Geometry check sheet. Reference: the model listing, model coordinates, mm. A direction names the side the tool comes from. Coordinates: 2 decimals unless noted, no trailing zeros. Loops run counter-clockwise (first coordinate to the right, second up) from the corner with the lowest first, then second, coordinate; pieces in that order, holes last.
Autodesk Inventor part; units mm, degrees
sketch "Эскиз1" plane through (0, 0, 0) normal (0, 0, 1) x (1, 0, 0)
  line L0 (-29.5, -27.5) -> (29.5, -27.5)
  line L1 (29.5, -27.5) -> (29.5, 27.5)
  line L2 (29.5, 27.5) -> (-29.5, 27.5)
  line L3 (-29.5, 27.5) -> (-29.5, -27.5)
  line L4 (-29.5, -27.5) -> (29.5, 27.5) construction
  line L5 (29.5, -27.5) -> (-29.5, 27.5) construction
  line L6 (0, -7.5) -> (0, -27.5) construction
  circle A0 centre (-21.05, 22.5) radius 1.5
  circle A1 centre (21.05, 22.5) radius 1.5
  line L7 (-21.05, 22.5) -> (21.05, 22.5)
  point P0 (0, 0)
  dimension "d0" = 59
  dimension "d1" = 55
  dimension "d3" = 20
  dimension "d4" = 3
  dimension "d7" = 42.1
  dimension "d8" = 8.45
  dimension "d13" = 5
extrude "Выдавливание1" add sketch "Эскиз1" along normal blind 4
sketch "Эскиз2" plane through (0, 0, 4) normal (0, 0, 1) x (1, 0, 0)
  line L0 (29.5, 27.5) -> (-29.5, 27.5)
  line L1 (-2.5247, 27.5) -> (-2.5247, 11.5)
  line L2 (2.5247, 27.5) -> (2.5247, 11.5)
  line L3 (-2.5247, 11.5) -> (2.5247, 11.5)
  point P0 (0, 0)
  dimension "d9" = 16
extrude "Выдавливание2" cut sketch "Эскиз2" against normal up to surface (4 mm away)
fillet "Сопряжение1" radius 2 4 edges at (2.5247, 11.5, 2) (-2.5247, 11.5, 2) (2.5247, 27.5, 2) (-2.5247, 27.5, 2)
sketch "Эскиз3" plane through (0, 0, 4) normal (0, 0, 1) x (1, 0, 0)
  line L0 (-29.5, 27.5) -> (-29.5, -27.5)
  line L1 (-29.5, -17.5) -> (-19.5, -17.5) construction
  line L2 (-19.5, -17.5) -> (-19.5, -27.5) construction
  line L3 (-29.5, -27.5) -> (29.5, -27.5)
  line L4 (-29.5, 27.5) -> (-29.5, -27.5)
  line L5 (-29.5, -27.5) -> (29.5, -27.5)
  line L6 (19.5, -27.5) -> (19.5, -17.5) construction
  line L7 (19.5, -17.5) -> (29.5, -17.5) construction
  line L8 (29.5, -27.5) -> (29.5, 27.5)
  arc A0 (-29.5, -17.5) -> (-19.5, -27.5) centre (-19.5, -17.5) ccw
  arc A1 (19.5, -27.5) -> (29.5, -17.5) centre (19.5, -17.5) ccw
  point P0 (0, 0)
extrude "Выдавливание3" cut sketch "Эскиз3" against normal up to surface (4 mm away)
properties part number "Скоба трубы"
(1) Draft check along Y on faces 1 (the cylindrical face through (-21, 21, 2)), 2 (the flat face through (0, 0, 4)), 3 (the flat face through (17, 27.5, 2)), 4 (the cylindrical face through (26.49, -24.65, 2.03)). Enter one of: +Y half, -Y half, draft (parallel to the pull), parting line (faces both ways), or undercut.
Findings:
face 1: undercut
face 2: draft
face 3: +Y half
face 4: -Y half
(2) Sectioned sample at B-B on y = 22.5. Record the cut outline in (x, z).
Findings:
outline: (-29.5, 0) - (-22.55, 0) - (-22.55, 4) - (-29.5, 4) - close; (-19.55, 0) - (-2.52, 0) - (-2.52, 4) - (-19.55, 4) - close; (2.52, 0) - (19.55, 0) - (19.55, 4) - (2.52, 4) - close; (22.55, 0) - (29.5, 0) - (29.5, 4) - (22.55, 4) - close
(3) Sectioned sample at C-C on y = 17. Record the cut outline in (x, z), and give its area (3 significant figures).
Findings:
outline: (-29.5, 0) - (-2.52, 0) - (-2.52, 4) - (-29.5, 4) - close; (2.52, 0) - (29.5, 0) - (29.5, 4) - (2.52, 4) - close
area: 216 mm2
(4) Gauge pin test, flat ends, axial feed: pin 1 Ø1.5 at (x, z) = (0, 2.5) entering from +Y; pin 2 Ø1.5 at (x, z) = (-23, 1.5) entering from -Y. Record the tip position at first contact, or that the pin passes through.
Findings:
pin 1: stops at y = 11.51
pin 2: stops at y = -27.11
(5) Scan lines: L1, parallel to X at y = 16, z = 1.8; L2, parallel to X at y = 12.5, z = 0.7; L3, parallel to Y at x = -21.05, z = 0.9. Record each from-to range of solid material in increasing order.
Findings:
L1: x = -29.5 to -2.52, 2.52 to 29.5
L2: x = -29.5 to -2.26, 2.26 to 29.5
L3: y = -27.38 to 21, 24 to 27.5
(6) Access from +Z, -Z, +X, -X, +Y, -Y to the whole of each face (thin tool, end or side, straight path). Record for faces 5 (the cylindrical face through (3.095, 26.899, 1.972)), 6 (the flat face through (-17, 27.5, 2)).
Findings:
face 5: +Z, -Z, +Y
face 6: +Z, -Z, +X, -X, +Y
(7) Sectioned sample at D-D on x = -21.05. Record the cut outline in (y, z).
Findings:
outline: (-27.38, 0) - (21, 0) - (21, 4) - (-27.38, 4) - close; (24, 0) - (27.5, 0) - (27.5, 4) - (24, 4) - close
(8) Sectioned sample at A-A on z = 3.1. Record the cut outline in (x, y).
Findings:
outline: (-29.5, -17.5) arc R10 ccw to (-19.5, -27.5) - (19.5, -27.5) arc R10 ccw to (29.5, -17.5) - (29.5, 27.5) - (4.52, 27.5) arc R2 ccw to (2.52, 25.5) - (2.52, 13.5) arc R2 cw to (0.52, 11.5) - (-0.52, 11.5) arc R2 cw to (-2.52, 13.5) - (-2.52, 25.5) arc R2 ccw to (-4.52, 27.5) - (-29.5, 27.5) - close; hole circle Ø3 at (-21.05, 22.5); hole circle Ø3 at (21.05, 22.5)
